Verification items for the finished model (mm, model axes). A direction names the side the tool comes from. Round coordinates to 2 decimals unless told otherwise and drop trailing zeros. Loops run counter-clockwise (first coordinate to the right, second up) from the corner with the lowest first, then second, coordinate; pieces in that order, holes last. Notation, with made-up numbers: (83.25, 88) -> (129.25, 88) arc R26 cw to (129.25, 105) -> close; hole circle Ø6 at (56, 64). An arc over 180 degrees is marked (long way). Write item = value, one per line.
```python
from build123d import *

# Parameters (mm, degrees)
SKETCH_R             = 1.6
PAD_DEPTH            = 8
POCKET_DEPTH         = 6
SKETCH001_W          = 18
SKETCH001_H          = 10
PAD001_DEPTH         = 8
POCKET001_DEPTH      = 34
POCKET001_DEPTH_BACK = 12
POCKET002_DEPTH      = 8.001


with BuildPart() as part:
    # Sketch → Pad (new body)
    with BuildSketch(Plane(origin=(0, 0, 34.387781), x_dir=(-1, 0, 0), z_dir=(0, 0, 1))):
        with BuildLine():
            Line((-25.159705, 9.979942), (-13.422916, 32.053632))
            ThreePointArc((34.079665, 6.796062), (19.106838, 35.934736), (-13.422916, 32.053632))
            Line((34.079665, 6.796062), (22.342876, -15.277628))
            Line((22.342876, -15.277628), (15.279295, -11.521855))
            Line((15.279295, -11.521855), (19.035067, -4.458275))
            Line((19.035067, -4.458275), (23.516593, 10.147407))
            Line((23.516593, 10.147407), (-4.73773, 25.170497))
            Line((-14.340352, 13.287751), (-4.73773, 25.170497))
            Line((-18.096124, 6.22417), (-14.340352, 13.287751))
            Line((-18.096124, 6.22417), (-25.159705, 9.979942))
        make_face()
        with Locations((-19.336552, 10.281427)):
            Circle(SKETCH_R, mode=Mode.SUBTRACT)
        with Locations((19.336552, -10.281427)):
            Circle(SKETCH_R, mode=Mode.SUBTRACT)
    extrude(amount=PAD_DEPTH)

    # Sketch004 → Pocket (cut)
    with BuildSketch(Plane(origin=(0, 0, 34.387781), x_dir=(-1, 0, 0), z_dir=(0, 0, -1))):
        with BuildLine():
            ThreePointArc((-10.535805, -28.111259), (14.805415, -27.844935), (29.196837, -6.985039))
            Line((23.510102, 7.970263), (29.196837, -6.985039))
            Line((23.510102, 7.970263), (33.765539, 13.423175))
            Line((33.765539, 13.423175), (24.376107, 31.082127))
            Line((24.376107, 31.082127), (-39.399197, -2.827804))
            Line((-39.399197, -2.827804), (-30.009766, -20.486756))
            Line((-30.009766, -20.486756), (-19.75433, -15.033844))
            Line((-19.75433, -15.033844), (-10.535805, -28.111259))
        make_face()
    extrude(amount=-POCKET_DEPTH, mode=Mode.SUBTRACT)

    # Sketch001 (on Face13 of Pad) → Pad001 (join)
    with BuildSketch(Plane(origin=(0, 0, 34.387781), x_dir=(-1, 0, 0), z_dir=(0, 0, -1))):
        with Locations((14, -27)):
            Rectangle(SKETCH001_W, SKETCH001_H)
    extrude(amount=-PAD001_DEPTH)

    # Sketch006 (on Face16 of Pad001) → Pocket001 (cut, two sides)
    with BuildSketch(Plane(origin=(0, -22, 34.387781), x_dir=(-1, 0, 0), z_dir=(0, 1, 0))) as pocket001_sk:
        Polygon((11.946699, 4.25), (15.053301, 4.25), (17.25, 6.446699), (17.25, 9.446699), (9.75, 9.446699), (9.75, 6.446699), align=None)
    extrude(amount=-POCKET001_DEPTH, mode=Mode.SUBTRACT)
    extrude(pocket001_sk.sketch, amount=POCKET001_DEPTH_BACK, mode=Mode.SUBTRACT)

    # Sketch007 (on Face29 of Pocket001) → Pocket002 (cut, through all)
    with BuildSketch(Plane(origin=(0, 0, 42.387781), x_dir=(-1, 0, 0), z_dir=(0, 0, 1))):
        Polygon((-3.522127, 23.490412), (21.597948, 23.490412), (22.751427, 9.520575), align=None)
    extrude(amount=-POCKET002_DEPTH, mode=Mode.SUBTRACT)


solid = part.part
```
(1) Sectioned sample at D-D, the plane y = 3. Record the cut outline in (x, z), and give its area (3 significant figures).
Filled sheet:
outline = (-28.87, 34.39) -> (-25.4, 34.39) -> (-25.4, 40.39) -> (-19.48, 40.39) -> (-19.48, 42.39) -> (-28.87, 42.39) -> close
area = 39.6 mm2
(2) Sectioned sample at A-A, the plane z = 37. Record the cut outline in (x, y).
Filled sheet:
outline = (-34.08, -6.8) arc R28.7 ccw to (13.42, -32.05) -> (21.87, -16.16) -> (19.75, -15.03) -> (10.54, -28.11) arc R27.54 cw to (-5, -30.89) -> (-5, -23.49) -> (-21.6, -23.49) -> (-21.72, -22) -> (-22.3, -22) arc R27.54 cw to (-29.2, -6.99) -> (-23.51, 7.97) -> (-25.63, 9.1) -> close
(3) Set-up check for faces 1 (the face through (-22.05, -18.03, 41.07)), 2 (the face through (20.829, -15.605, 37.346)), 3 (the face through (-26.314, 0.597, 37.346)), 4 (the face through (-10.833, -31.135, 39.752)): record each of +Z, -Z, +X, -X, +Y, -Y from which the full face is reachable in a straight line by a thin tool's end or side.
Filled sheet:
face_1 = +Z, -Z
face_2 = -Z, +X, +Y
face_3 = -Z, +X
face_4 = +Z, +Y, -Y
(4) Material ranges on probe 1 along Y at (x, z) = (-18, 41); probe 2 along Z at (x, y) = (-24, 10.5); probe 3 along X at (y, z) = (11.5, 41.5), recorded low to high. Write a range as from..to.
Filled sheet:
probe_1 = -36.49..-23.49, 6.4..9.4, 11.16..12.97
probe_2 = 40.39..42.39
probe_3 = -24.35..-20.37, -18.3..-15.29
(5) Go/stop test with flat-tipped pins: pin 1 Ø1.5 at (y, z) = (-28.5, 39.5) entering from -X; pin 2 Ø4 at (y, z) = (-3.5, 36) entering from +X; pin 3 Ø3.5 at (x, y) = (-19.34, 10.28) entering from -Z. Record where each tip stops, or that it passes through.
Filled sheet:
pin_1 = -28.64
pin_2 = -27.11
pin_3 = 40.39
(6) Draft check along Y on faces 5 (the face through (16.245, -9.707, 41.374)), 6 (the face through (-21.244, -2.742, 41.374)), 7 (the face through (7, -27, 42.388)). Enter one of: released by +Y, released by -Y, zero draft, split by the parting line, or undercut.
Filled sheet:
face_5 = released by +Y
face_6 = undercut
face_7 = zero draft
(7) Sectioned sample at C-C, the plane x = 2.5. Record the cut outline in (y, z), and give its area (3 significant figures).
Filled sheet:
outline = (-38.12, 34.39) -> (-30.72, 34.39) -> (-30.72, 40.39) -> (-23.98, 40.39) -> (-23.98, 42.39) -> (-38.12, 42.39) -> close
area = 72.7 mm2
(8) Sectioned sample at B-B, the plane y = -33. Record the cut outline in (x, z).
Filled sheet:
outline = (-23.57, 34.39) -> (12.3, 34.39) -> (12.3, 42.39) -> (-9.75, 42.39) -> (-9.75, 40.83) -> (-11.95, 38.64) -> (-15.05, 38.64) -> (-17.25, 40.83) -> (-17.25, 42.39) -> (-23.57, 42.39) -> close
